```python
from build123d import *

# Parameters (mm, degrees)
F0_R     = 60
F0_R_2   = 49.05
F1_DEPTH = 3
F2_R     = 1.5
F2_R_2   = 2
F3_DEPTH = 3.001
F4_R     = 2


with BuildPart() as f1:
    # F0 (on Front) → F1 (new body)
    with BuildSketch(Plane.XZ):
        Circle(F0_R)
        Circle(F0_R_2, mode=Mode.SUBTRACT)
    extrude(amount=F1_DEPTH)

    # F2 (on face) → F3 (cut, through all)
    with BuildSketch(Plane.XZ.offset(3)):
        with Locations((-52.5, 0)):
            Circle(F2_R)
        with Locations((0, 52.5)):
            Circle(F2_R)
        with Locations((52.5, 0)):
            Circle(F2_R)
        with Locations((0, -52.5)):
            Circle(F2_R)
        Polygon((59.6694861809, 25.7983026362), (40.3142099748, 17.7810847282), (40.6968934071, 16.8572051957), (41.0795768395, 15.9333256632), (60.4348530456, 23.9505435712), (60.0521696132, 24.8744231037), align=None)
        with Locations((-38.8908729653, 38.8908729653)):
            Circle(F2_R_2)
        with Locations((-38.8908729653, -38.8908729653)):
            Circle(F2_R_2)
        with Locations((38.8908729653, -38.8908729653)):
            Circle(F2_R_2)
        with Locations((38.8908729653, 38.8908729653)):
            Circle(F2_R_2)
    extrude(amount=-F3_DEPTH, mode=Mode.SUBTRACT)

    # F4
    f4_edges = [f1.edges().sort_by_distance(p)[0] for p in [
        (55.042389, -1.5, 23.881696),
        (55.807756, -1.5, 22.033937),
        (44.924189, -1.5, 19.690601),
        (45.689556, -1.5, 17.842841),
    ]]
    fillet(f4_edges, radius=F4_R)


solid = f1.part
```
The listing builds one solid part. Answer for the finished solid, in the listing's coordinates (mm). A direction names the side the tool comes from. Give positions to 0.01 mm unless a question says otherwise; leave off trailing zeros. Write each loop counter-clockwise with the first axis right and the second up, starting at its lowest first coordinate (ties: lowest second). Pieces come first, ordered by that corner, then holes. Notation, with made-up numbers: (42, 74.25) - (62, 74.25) arc R35 cw to (62, 109.25) - close; hole circle Ø8 at (-28, 42.5). An arc over 180 degrees is marked (long way). Use one line per item in the form item = value. Start each with the question number.
1) Flat-ended cylindrical pins translate along their axes: pin 1 Ø3.5 at (x, z) = (38.89, 38.89) entering from +Y; pin 2 Ø5 at (x, z) = (0, -52.5) entering from -Y; pin 3 Ø1.5 at (x, y) = (-33.5, -1) entering from -Z; pin 4 Ø1.5 at (x, y) = (36.5, -2.5) entering from +Z. Find the tip coordinate at first contact, or state that the pin passes through.
2) A tool of negligible diameter and unlimited length cuts with its end or side. For faces 4 (the face through (49.96, -1.521, 21.777)), 5 (the face through (54.224, -1.479, 24.199)), from which of +Z, -Z, +X, -X, +Y, -Y can it reach the whole face along a straight path? Write none if from no direction.
3) Find section C-C on x = 42.5. Determine the outline of the cut face in (y, z), plus the area to 3 significant figures.
4) Find section D-D on y = -1. Count the separate pieces of the cut face and the enclosed holes in it, plus the area to 3 significant figures.
5) Find section A-A on z = 0. Determine the outline of the cut face in (x, y).
6) The mould has two halves that part along Z. Classify faces 1 (the face through (50.636, -1.521, 19.892)), 2 (the face through (-9, 0, -49)), 3 (the face through (-56.374, -1.479, -20.542)): pulls with the +Z half, pulls with the -Z half, needs draft (parallel to the pull), parting line crosses it, or undercut.
7) Consider line 1 along Z through (x, y) = (0, -2); line 2 along Z through (x, y) = (-40.5, -1.65); line 3 along Z through (x, y) = (-52.5, -1.45). Determine where each line is inside the solid, lowest interval first. Write a range as from..to.
8) Find section B-B on x = 0. Determine the outline of the cut face in (y, z), plus the area to 3 significant figures.
Geometry results:
q1.pin_1 = through
q1.pin_2 = -3
q1.pin_3 = -50.27
q1.pin_4 = 48.19
q2.face_4 = +Y, -Y
q2.face_5 = +X, +Y, -Y
q3.outline = (-3, -42.35) - (0, -42.35) - (0, -24.49) - (-3, -24.49) - close; (-3, 24.49) - (0, 24.49) - (0, 42.35) - (-3, 42.35) - close
q3.area = 107 mm2
q4.separate_pieces = 1
q4.enclosed_holes = 8
q4.area = 3,650 mm2
q5.outline = (-60, -3) - (-54, -3) - (-54, 0) - (-60, 0) - close; (-51, -3) - (-49.05, -3) - (-49.05, 0) - (-51, 0) - close; (49.05, -3) - (51, -3) - (51, 0) - (49.05, 0) - close; (54, -3) - (60, -3) - (60, 0) - (54, 0) - close
q6.face_1 = undercut
q6.face_2 = needs draft
q6.face_3 = parting line crosses it
q7.line_1 = -60..-54, -51..-49.05, 49.05..51, 54..60
q7.line_2 = -44.27..-40.08, -37.7..-27.67, 27.67..37.7, 40.08..44.27
q7.line_3 = -29.05..-1.5, 1.5..29.05
q8.outline = (-3, -60) - (0, -60) - (0, -54) - (-3, -54) - close; (-3, -51) - (0, -51) - (0, -49.05) - (-3, -49.05) - close; (-3, 49.05) - (0, 49.05) - (0, 51) - (-3, 51) - close; (-3, 54) - (0, 54) - (0, 60) - (-3, 60) - close
q8.area = 47.7 mm2
